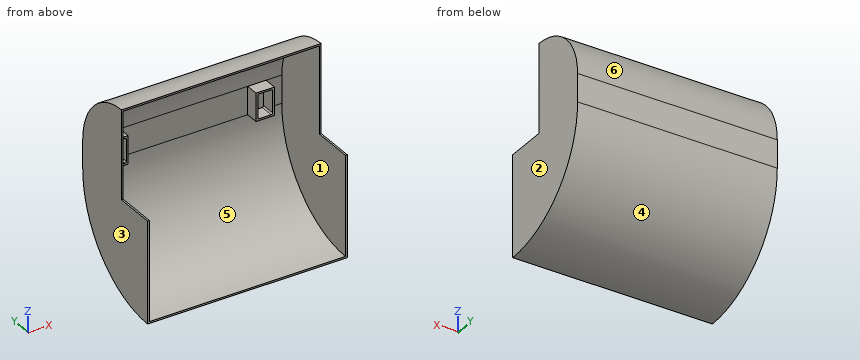
from build123d import *

# Parameters (mm, degrees)
SKETCH1_W                = 33.3375
SKETCH1_H                = 50.8
SKETCH1_W_2              = 26.9875
SKETCH1_H_2              = 44.45
BOSS_EXTRUDE1_DEPTH      = 25.4
FILLET2_R                = 2.54
SKETCH2_W                = 33.3375
SKETCH2_H                = 50.8
BOSS_EXTRUDE2_DEPTH      = 1.5875
SKETCH1_5_W              = 33.3375
SKETCH1_5_H              = 50.8
BOSS_EXTRUDE3_DEPTH      = 26.9875
SKETCH1_6_W              = 26.9875
SKETCH1_6_H              = 44.45
CUT_EXTRUDE1_DEPTH       = 25.4
FILLET4_R                = 2.54
BOSS_EXTRUDE4_DEPTH      = 31.75
BOSS_EXTRUDE4_DEPTH_BACK = 330.2
SKETCH6_W                = 231.775
SKETCH6_H                = 3.175
BOSS_EXTRUDE5_DEPTH      = 50.8
BOSS_EXTRUDE6_DEPTH      = 31.75
BOSS_EXTRUDE6_DEPTH_BACK = 330.2
BOSS_EXTRUDE7_START      = -3.175
BOSS_EXTRUDE7_DEPTH      = 3.175
SKETCH10_W               = 50.8
SKETCH10_H               = 3.2258
BOSS_EXTRUDE8_DEPTH      = 31.75
SKETCH11_W               = 3.175
SKETCH11_H               = 180.9242
BOSS_EXTRUDE9_DEPTH      = 50.8
BOSS_EXTRUDE12_START     = -3.175
BOSS_EXTRUDE12_DEPTH     = 3.175
SKETCH14_W               = 50.8
SKETCH14_H               = 3.2258
BOSS_EXTRUDE13_DEPTH     = 31.75
BOSS_EXTRUDE14_DEPTH     = 3.175
SKETCH17_W               = 3.175
SKETCH17_H               = 50.8
BOSS_EXTRUDE15_DEPTH     = 106.8324
BOSS_EXTRUDE16_DEPTH     = 3.175
CUT_EXTRUDE2_REACH       = 452.066
SKETCH21_W               = 50.8
SKETCH21_H               = 74.0918


with BuildPart() as part:
    # Sketch1 → Boss-Extrude1 (new body)
    with BuildSketch(Plane(origin=(0, 0, 0), x_dir=(1, 0, 0), z_dir=(0, 1, 0))):
        with Locations((0.204179282, 6.901311315)):
            Rectangle(SKETCH1_W, SKETCH1_H)
        with Locations((0.204179282, 6.901311315)):
            Rectangle(SKETCH1_W_2, SKETCH1_H_2, mode=Mode.SUBTRACT)
    extrude(amount=BOSS_EXTRUDE1_DEPTH)

    # Fillet2
    fillet2_edges = [part.edges().sort_by_distance(p)[0] for p in [
        (13.697929282, 12.7, 15.323688685),
        (13.697929282, 12.7, -29.126311315),
        (-13.289570718, 12.7, -29.126311315),
        (-13.289570718, 12.7, 15.323688685),
    ]]
    fillet(fillet2_edges, radius=FILLET2_R)

    # Sketch2 → Boss-Extrude2 (add)
    with BuildSketch(Plane(origin=(0, 25.4, 0), x_dir=(1, 0, 0), z_dir=(0, 1, 0))):
        with Locations((0.204179282, 6.901311315)):
            Rectangle(SKETCH2_W, SKETCH2_H)
    extrude(amount=BOSS_EXTRUDE2_DEPTH)



with BuildPart() as body_2:
    # Sketch1<5> → Boss-Extrude3 (new body)
    with BuildSketch(Plane(origin=(0, 0, 0), x_dir=(1, 0, 0), z_dir=(0, 1, 0))):
        with Locations((-264.908320718, 6.901311315)):
            Rectangle(SKETCH1_5_W, SKETCH1_5_H)
    extrude(amount=BOSS_EXTRUDE3_DEPTH)

    # Sketch1<6> → Cut-Extrude1 (cut)
    with BuildSketch(Plane(origin=(0, 0, 0), x_dir=(1, 0, 0), z_dir=(0, 1, 0))):
        with Locations((-264.908320718, 6.901311315)):
            Rectangle(SKETCH1_6_W, SKETCH1_6_H)
    extrude(amount=CUT_EXTRUDE1_DEPTH, mode=Mode.SUBTRACT)

    # Fillet4
    fillet4_edges = [body_2.edges().sort_by_distance(p)[0] for p in [
        (-251.414570718, 12.7, 15.323688685),
        (-251.414570718, 12.7, -29.126311315),
        (-278.402070718, 12.7, -29.126311315),
        (-278.402070718, 12.7, 15.323688685),
    ]]
    fillet(fillet4_edges, radius=FILLET4_R)


with BuildPart() as part_1:
    add(part.part)

    add(body_2.part)  # Boss-Extrude4 merges body 2
    # Sketch4 → Boss-Extrude4 (add, two sides: drawn at the far end of the back side and taken through both)
    with BuildSketch(Plane(origin=(16.872929282, 0, 0), x_dir=(0, 0, -1), z_dir=(1, 0, 0)).offset(-BOSS_EXTRUDE4_DEPTH_BACK)):
        with BuildLine():
            ThreePointArc((32.301311315, 23.8125), (160.269961041, -29.193850275), (213.276311315, -157.1625))
            Line((213.276311315, -157.1625), (216.451311315, -157.1625))
            ThreePointArc((216.451311315, -157.1625), (162.515025071, -26.948786244), (32.301311315, 26.9875))
            Line((32.301311315, 26.9875), (32.301311315, 23.8125))
        make_face()
    extrude(amount=BOSS_EXTRUDE4_DEPTH + BOSS_EXTRUDE4_DEPTH_BACK)

    # Sketch6 → Boss-Extrude5 (add, through all)
    with BuildSketch(Plane.XY.offset(-32.301311315)):
        with Locations((-132.352070718, 25.4)):
            Rectangle(SKETCH6_W, SKETCH6_H)
    extrude(amount=BOSS_EXTRUDE5_DEPTH)

    # Sketch7 → Boss-Extrude6 (add, two sides: drawn at the far end of the back side and taken through both)
    with BuildSketch(Plane(origin=(16.872929282, 0, 0), x_dir=(0, 0, -1), z_dir=(1, 0, 0)).offset(-BOSS_EXTRUDE6_DEPTH_BACK)):
        with BuildLine():
            Line((-18.498688685, 23.7617), (-18.498688685, 26.9875))
            ThreePointArc((-18.498688685, 26.9875), (-96.32158823, -5.247800455), (-128.556888685, -83.0707))
            Line((-128.556888685, -83.0707), (-125.331088685, -83.0707))
            ThreePointArc((-125.331088685, -83.0707), (-94.040603175, -7.52878551), (-18.498688685, 23.7617))
        make_face()
    extrude(amount=BOSS_EXTRUDE6_DEPTH + BOSS_EXTRUDE6_DEPTH_BACK)

    # Sketch9 → Boss-Extrude7 (add)
    with BuildSketch(Plane(origin=(48.622929282, 0, 0), x_dir=(0, 0, -1), z_dir=(1, 0, 0)).offset(BOSS_EXTRUDE7_START)):
        with BuildLine():
            Line((32.301311315, 23.8125), (32.301311315, -157.1625))
            Line((32.301311315, -157.1625), (213.276311315, -157.1625))
            ThreePointArc((213.276311315, -157.1625), (160.269961041, -29.193850275), (32.301311315, 23.8125))
        make_face()
    extrude(amount=BOSS_EXTRUDE7_DEPTH)

    # Sketch10 → Boss-Extrude8 (add)
    with BuildSketch(Plane(origin=(16.872929282, 0, 0), x_dir=(0, 0, -1), z_dir=(1, 0, 0))):
        with Locations((6.901311315, 25.3746)):
            Rectangle(SKETCH10_W, SKETCH10_H)
    extrude(amount=BOSS_EXTRUDE8_DEPTH)

    # Sketch11 → Boss-Extrude9 (add)
    with BuildSketch(Plane.XY.offset(-32.301311315)):
        with Locations((47.035429282, -66.7004)):
            Rectangle(SKETCH11_W, SKETCH11_H)
    extrude(amount=BOSS_EXTRUDE9_DEPTH)

    # Sketch13 → Boss-Extrude12 (add)
    with BuildSketch(Plane(origin=(48.622929282, 0, 0), x_dir=(0, 0, -1), z_dir=(1, 0, 0)).offset(BOSS_EXTRUDE12_START)):
        with BuildLine():
            Line((-125.331088685, -83.0707), (-18.498688685, -83.0707))
            Line((-18.498688685, -83.0707), (-18.498688685, 23.7617))
            ThreePointArc((-18.498688685, 23.7617), (-94.040603175, -7.52878551), (-125.331088685, -83.0707))
        make_face()
    extrude(amount=BOSS_EXTRUDE12_DEPTH)

    # Sketch14 → Boss-Extrude13 (add)
    with BuildSketch(Plane.ZY.offset(281.577070718)):
        with Locations((-6.901311315, 25.3746)):
            Rectangle(SKETCH14_W, SKETCH14_H)
    extrude(amount=BOSS_EXTRUDE13_DEPTH)

    # Sketch15 → Boss-Extrude14 (add)
    with BuildSketch(Plane.ZY.offset(313.327070718)):
        with BuildLine():
            Line((-213.276311315, -157.1625), (-32.301311315, -157.1625))
            Line((-32.301311315, -157.1625), (-32.301311315, 23.8125))
            ThreePointArc((-32.301311315, 23.8125), (-160.269961041, -29.193850275), (-213.276311315, -157.1625))
        make_face()
    extrude(amount=-BOSS_EXTRUDE14_DEPTH)

    # Sketch17 → Boss-Extrude15 (add)
    with BuildSketch(Plane.XZ.offset(-23.7617)):
        with Locations((-311.739570718, -6.901311315)):
            Rectangle(SKETCH17_W, SKETCH17_H)
    extrude(amount=BOSS_EXTRUDE15_DEPTH)

    # Sketch18 → Boss-Extrude16 (add)
    with BuildSketch(Plane.ZY.offset(313.327070718)):
        with BuildLine():
            Line((18.498688685, 23.7617), (18.498688685, -83.0707))
            Line((18.498688685, -83.0707), (125.331088685, -83.0707))
            ThreePointArc((125.331088685, -83.0707), (94.040603175, -7.52878551), (18.498688685, 23.7617))
        make_face()
    extrude(amount=-BOSS_EXTRUDE16_DEPTH)

    # Sketch21 → Cut-Extrude2 (cut, up to next)
    with BuildSketch(Plane(origin=(48.622929282, 0, 0), x_dir=(0, 0, -1), z_dir=(1, 0, 0)), mode=Mode.PRIVATE) as cut_extrude2_sk1:
        with Locations((6.901311315, -120.1166)):
            Rectangle(SKETCH21_W, SKETCH21_H)
    cut_extrude2_tool1 = extrude(cut_extrude2_sk1.sketch, amount=-CUT_EXTRUDE2_REACH, mode=Mode.PRIVATE) & part_1.part
    add(cut_extrude2_tool1.solids().sort_by_distance((48.622929, -120.1166, -6.901311))[0], mode=Mode.SUBTRACT)


solid = part_1.part
Source: CAD feature listing. Evaluate the final solid. Frame: model axes, mm. Face numbers are marked on the shaded views. A direction names the side the tool comes from. Coordinates: 2 decimals unless noted, no trailing zeros. Order: outer loops, then holes, each group sorted by start corner. A loop starts at its lowest first (then second) coordinate and runs counter-clockwise, first axis right, second up.
Item 1: Cut plane C-C (z = -18). Return loops of the section in (x, y).
Output values:
outline: (-313.33, -83.07) - (-310.15, -83.07) - (-310.15, 23.76) - (-281.58, 23.76) - (-281.58, 0) - (-278.4, 0) - (-278.4, 25.4) - (-251.41, 25.4) - (-251.41, 0) - (-248.24, 0) - (-248.24, 23.81) - (-16.46, 23.81) - (-16.46, 0) - (-13.29, 0) - (-13.29, 25.4) - (13.7, 25.4) - (13.7, 0) - (16.87, 0) - (16.87, 23.76) - (45.45, 23.76) - (45.45, -83.07) - (48.62, -83.07) - (48.62, 26.99) - (-313.33, 26.99) - close
Item 2: Set-up query: the marked faces 5 and 6. Return all of +Z, -Z, +X, -X, +Y, -Y with unobstructed straight access to the full face (end or side cutting, diameter ignored); none if empty.
Output values:
face 5: -Y
face 6: +Z, +X, -X, +Y
Item 3: Material intervals for line 1 (X direction, y = 18.5, z = 37.5); line 2 (Y direction, x = -274.5, z = -16); line 3 (Y direction, x = -14.5, z = -22.5), sorted ascending.
Output values:
line 1: x = -313.33 to -310.15, 45.45 to 48.62
line 2: y = 25.4 to 26.99
line 3: y = 0 to 26.99
Item 4: First-contact query: P1, Ø10, axis at x = -35.5, y = -29.5, coming from the -Z side; P2, Ø1.5, axis at x = -118, y = -20.5, coming from the +Z side; P3, Ø10, axis at x = -3.5, z = -9.5, coming from the -Y side; P4, Ø4, axis at x = -26.5, y = -84.5, coming from the +Z side. Flat tips, straight axial feed; report the tip coordinate or a pass-through.
Output values:
P1: stops at z = -169.65
P2: stops at z = 109.55
P3: stops at y = 25.4
P4: stops at z = 128.56
Item 5: Pull-direction query (X, two-part tool) for the marked faces 1, 2, 3 and 4; classes: pulls with the +X half, pulls with the -X half, needs draft (parallel to the pull), parting line crosses it, or undercut.
Output values:
face 1: undercut
face 2: pulls with the +X half
face 3: pulls with the -X half
face 4: needs draft
Item 6: Cut plane B-B (y = -61). Return loops of the section in (x, z).
Output values:
outline: (-313.33, -189.35) - (48.62, -189.35) - (48.62, 126.32) - (-313.33, 126.32) - close; hole (-310.15, -185.61) - (45.45, -185.61) - (45.45, 123.03) - (-310.15, 123.03) - close
Item 7: Cut plane D-D (y = -139). Return loops of the section in (x, z), plus the area to 3 significant figures.
Output values:
outline: (-313.33, -215.55) - (48.62, -215.55) - (48.62, -32.3) - (45.45, -32.3) - (45.45, -212.36) - (-310.15, -212.36) - (-310.15, -32.3) - (-313.33, -32.3) - close
area: 2,300 mm2
